```python
from build123d import *

# Parameters (mm, degrees)
F0_W     = 85.09
F0_H     = 95.25
F1_DEPTH = 6.35
F2_R     = 1.905
F2_W     = 6.35
F2_H     = 12.7
F2_H_2   = 6.35
F3_DEPTH = 6.351
F4_DEPTH = 132


# Not quite as in the source:
# - an extrude ends at something that could not be found from the text; its depth is read off the source's solid


with BuildPart() as f1:
    # F0 (on Top) → F1 (new body)
    with BuildSketch(Plane.XY):
        Rectangle(F0_W, F0_H)
    extrude(amount=F1_DEPTH)

    # F2 (on Top) → F3 (cut, through all)
    with BuildSketch(Plane.XY):
        with Locations((-17.145, -25.4)):
            Circle(F2_R)
        with Locations((-17.145, 25.4)):
            Circle(F2_R)
        with Locations((8.255, -25.4)):
            Rectangle(F2_W, F2_H)
        with Locations((8.255, 34.925)):
            Rectangle(F2_W, F2_H_2)
        with Locations((8.255, 25.4)):
            Rectangle(F2_W, F2_H)
        with Locations((8.255, 15.875)):
            Rectangle(F2_W, F2_H_2)
        with Locations((27.305, 25.4)):
            Rectangle(F2_W, F2_H)
        with Locations((27.305, 34.925)):
            Rectangle(F2_W, F2_H_2)
        with Locations((27.305, 15.875)):
            Rectangle(F2_W, F2_H_2)
        with Locations((27.305, -25.4)):
            Rectangle(F2_W, F2_H)
        with Locations((17.78, 34.925)):
            Rectangle(F2_W, F2_H_2)
        with Locations((17.78, 25.4)):
            Rectangle(F2_W, F2_H)
        with Locations((17.78, 15.875)):
            Rectangle(F2_W, F2_H_2)
        with Locations((17.78, -25.4)):
            Rectangle(F2_W, F2_H)
    extrude(amount=F3_DEPTH, mode=Mode.SUBTRACT)

    # F2 (on Top) → F4 (cut, through all)
    with BuildSketch(Plane.XY):
        with Locations((-17.145, -25.4)):
            Circle(F2_R)
        with Locations((-17.145, 25.4)):
            Circle(F2_R)
        with Locations((8.255, -25.4)):
            Rectangle(F2_W, F2_H)
        with Locations((8.255, 34.925)):
            Rectangle(F2_W, F2_H_2)
        with Locations((8.255, 25.4)):
            Rectangle(F2_W, F2_H)
        with Locations((8.255, 15.875)):
            Rectangle(F2_W, F2_H_2)
        with Locations((27.305, 25.4)):
            Rectangle(F2_W, F2_H)
        with Locations((27.305, 34.925)):
            Rectangle(F2_W, F2_H_2)
        with Locations((27.305, 15.875)):
            Rectangle(F2_W, F2_H_2)
        with Locations((27.305, -25.4)):
            Rectangle(F2_W, F2_H)
        with Locations((17.78, 34.925)):
            Rectangle(F2_W, F2_H_2)
        with Locations((17.78, 25.4)):
            Rectangle(F2_W, F2_H)
        with Locations((17.78, 15.875)):
            Rectangle(F2_W, F2_H_2)
        with Locations((17.78, -25.4)):
            Rectangle(F2_W, F2_H)
    extrude(amount=-F4_DEPTH, mode=Mode.SUBTRACT)


solid = f1.part
```
Part model, mm, in its own coordinate system. A direction names the side the tool comes from. Round coordinates to 2 decimals unless told otherwise and drop trailing zeros. Write each loop counter-clockwise with the first axis right and the second up, starting at its lowest first coordinate (ties: lowest second). Pieces come first, ordered by that corner, then holes. Notation, with made-up numbers: M 86,-34.5 L 139,-34.5 A35 cw 139,-0.5 Z; hole C -13.5,78 d7. An arc over 180 degrees is marked long. Answer as CSV lines item,"result". Start each with the question number.
1) Band-saw the part on C-C (z = 2.5). Count the separate pieces of the cut face and the enclosed holes in it, then the cut area to 3 significant figures.
2) Band-saw the part on B-B (y = 21). List the corners of the cut face in (x, z) (3 decimals), then the cut area to 3 significant figures.
3) Which spindle directions (+Z, -Z, +X, -X, +Y, -Y) get a long thin tool onto all of the face, cutting with end or side? Do faces 4 (the face through (-1, 47.625, 3)), 5 (the face through (8, -19.05, 3)). Say none if no direction does.
4) Mould opens along X. For faces 1 (the face through (-42.545, -1, 3)), 2 (the face through (42.545, -1, 3)), 3 (the face through (20.955, 25, 3)) say: +X half, -X half, draft (parallel to the pull), parting line (faces both ways), or undercut.
5) Band-saw the part on A-A (y = -25.4). List the corners of the cut face in (x, z) (3 decimals), then the cut area to 3 significant figures.
6) Drill centre lines: L1, parallel to X at y = 25.4, z = 2 (3 decimals); L2, parallel to X at y = 34.5, z = 2.25 (3 decimals); L3, parallel to Y at x = 25.5, z = 2.5 (3 decimals). Where is each one in solid material? Low to high.
Worked out:
1,separate pieces,"1"
1,enclosed holes,"8"
1,area,"7,360 mm²"
2,outline,"M -42.545,0 L 5.08,0 L 5.08,6.35 L -42.545,6.35 Z; M 11.43,0 L 14.605,0 L 14.605,6.35 L 11.43,6.35 Z; M 20.955,0 L 24.13,0 L 24.13,6.35 L 20.955,6.35 Z; M 30.48,0 L 42.545,0 L 42.545,6.35 L 30.48,6.35 Z"
2,area,"419 mm²"
3,face 4,"+Z, -Z, +X, -X, +Y"
3,face 5,"+Z, -Z"
4,face 1,"-X half"
4,face 2,"+X half"
4,face 3,"undercut"
5,outline,"M -42.545,0 L -19.05,0 L -19.05,6.35 L -42.545,6.35 Z; M -15.24,0 L 5.08,0 L 5.08,6.35 L -15.24,6.35 Z; M 11.43,0 L 14.605,0 L 14.605,6.35 L 11.43,6.35 Z; M 20.955,0 L 24.13,0 L 24.13,6.35 L 20.955,6.35 Z; M 30.48,0 L 42.545,0 L 42.545,6.35 L 30.48,6.35 Z"
5,area,"395 mm²"
6,L1,"-42.545 to -19.05, -15.24 to 5.08, 11.43 to 14.605, 20.955 to 24.13, 30.48 to 42.545"
6,L2,"-42.545 to 5.08, 11.43 to 14.605, 20.955 to 24.13, 30.48 to 42.545"
6,L3,"-47.625 to -31.75, -19.05 to 12.7, 38.1 to 47.625"
